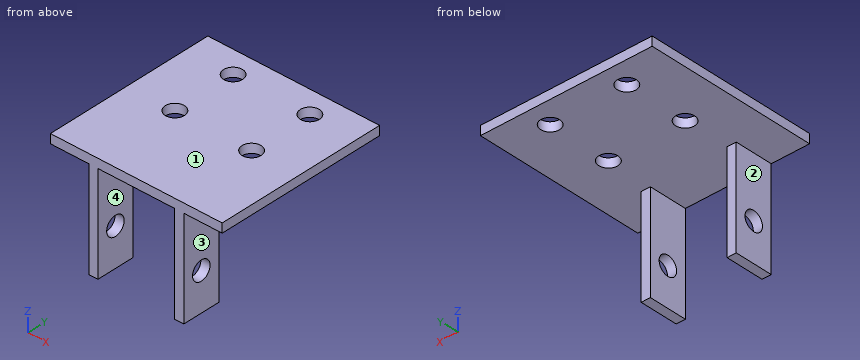
Autodesk Fusion 360 part; units mm, degrees
sketch "Sketch1" plane through (0, 0, 0) normal (0, 0, 1) x (1, 0, 0)
  line L0 (-13.45, 12) -> (31.55, 12)
  line L1 (31.55, 12) -> (31.55, -33)
  line L2 (31.55, -33) -> (-13.45, -33)
  line L3 (-13.45, -33) -> (-13.45, 12)
  line L4 (-3.4, -33) -> (-1, -33)
  line L5 (-1, -33) -> (-1, -23)
  line L6 (-1, -23) -> (-3.4, -23)
  line L7 (-3.4, -23) -> (-3.4, -33)
  line L8 (19.1, -23) -> (19.1, -33)
  line L9 (21.5, -23) -> (19.1, -23)
  line L10 (21.5, -33) -> (21.5, -23)
  line L11 (19.1, -33) -> (21.5, -33)
  circle A0 centre (-1, 5.65) radius 2.5
  circle A1 centre (-1, 5.65) radius 7.65
  circle A2 centre (19.1, 5.65) radius 7.65
  circle A3 centre (19.1, 5.65) radius 2.5
  circle A4 centre (-1, -11) radius 2.5
  circle A5 centre (19.1, -11) radius 2.5
  circle A6 centre (-1, -11) radius 9
  circle A7 centre (19.1, -11) radius 9
  dimension "d1" = 45
  dimension "d2" = 45
  dimension "d3" = 10
  dimension "d4" = 2.4
  dimension "d5" = 10.05
  dimension "d7" = 2.4
  dimension "d8" = 20.1
  dimension "d9" = 5
  dimension "d10" = 6.35
  dimension "d11" = 15.3
  dimension "d13" = 5
  dimension "d14" = 15.3
  dimension "d15" = 20.1
  dimension "d16" = 12.45
  dimension "d25" = 5
  dimension "d26" = 5
  dimension "d27" = 20.1
  dimension "d28" = 12.45
  dimension "d31" = 18
  dimension "d32" = 18
extrude "Extrude1" add sketch "Sketch1" along normal blind 2.4 contours A7 | A6 | L0 L1 L2 L3 L5 L6 L7 L8 L9 L10 A1 A2 | L0 A1 | L2 L4 L5 L6 L7 | L0 A2 | L2 L8 L9 L10 L11 | A4 | A5 picked at (-1.0623, 10.7143) picked at (19.0377, 10.7143)
extrude "Extrude2" add sketch "Sketch1" against normal blind 26 contours L2 L4 L5 L6 L7 | L2 L8 L9 L10 L11
sketch "Sketch2" plane through (21.5, 0, 0) normal (1, 0, 0) x (0, 1, 0)
  line L0 (-23, 0) -> (-33, 0)
  line L1 (-33, 0) -> (-33, -26)
  line L2 (-33, -26) -> (-23, -26)
  line L3 (-23, -26) -> (-23, 0)
  circle A0 centre (-28, -16) radius 2.5
  dimension "d21" = 5
  dimension "d22" = 10
extrude "Extrude3" cut sketch "Sketch2" against normal blind 30 contours A0
extrude "Extrude4" cut sketch "Sketch1" along normal blind 3 contours A4 | A5
Geometry: final body of the model. Coordinates: model frame, mm. Face numbers are marked on the shaded views. Round coordinates to 2 decimals unless told otherwise and drop trailing zeros. Write each loop counter-clockwise with the first axis right and the second up, starting at its lowest first coordinate (ties: lowest second). Pieces come first, ordered by that corner, then holes. Notation, with made-up numbers: M -16,-18.5 L -6,-18.5 A25 ccw -6,9.5 Z; hole C -32,31 d2. An arc over 180 degrees is marked long. Answer in a Markdown table with one row per item. Add a question column.
(1) Cut plane C-C, the plane z = -16. Return the cut outline in (x, y).
(2) Ray query, L1, parallel to X at y = -11, z = 1.8; L2, parallel to Y at x = 19.1, z = 0.7; L3, parallel to Z at x = -2.05, y = -28. Return the intervals inside material, ascending.
(3) Cut plane D-D, the plane y = -12.5. Return the cut outline in (x, z).
(4) Contact query for flat-ended pins moving along their axis: pin 1 (6 mm diameter, centred on x = -1, y = -11, fed in from -Z); pin 2 (8 mm diameter, centred on y = -28, z = -16, fed in from +X); pin 3 (6 mm diameter, centred on y = -28, z = -16, fed in from -X); pin 4 (4 mm diameter, centred on x = 19.1, y = -11, fed in from +Z). Output: stop coordinate, or through.
(5) Cut plane B-B, the plane z = -7.75. Return the cut outline in (x, y), then the cut area to 3 significant figures.
(6) Draft query along X for the marked faces 1, 2, 3 and 4. Return one class per face: pulls with the +X half, pulls with the -X half, needs draft (parallel to the pull), parting line crosses it, or undercut.
(7) Cut plane A-A, the plane y = -28. Return the cut outline in (x, z), then the cut area to 3 significant figures.
Established:
| question | item | result |
|---|---|---|
| 1 | outline | M -3.4,-33 L -1,-33 L -1,-30.5 L -3.4,-30.5 Z; M -3.4,-25.5 L -1,-25.5 L -1,-23 L -3.4,-23 Z; M 19.1,-33 L 21.5,-33 L 21.5,-30.5 L 19.1,-30.5 Z; M 19.1,-25.5 L 21.5,-25.5 L 21.5,-23 L 19.1,-23 Z |
| 2 | L1 | -13.45 to -3.5, 1.5 to 16.6, 21.6 to 31.55 |
| 2 | L2 | -33 to -13.5, -8.5 to 3.15, 8.15 to 12 |
| 2 | L3 | -26 to -18.5, -13.5 to 2.4 |
| 3 | outline | M -13.45,0 L -3,0 L -3,2.4 L -13.45,2.4 Z; M 1,0 L 17.1,0 L 17.1,2.4 L 1,2.4 Z; M 21.1,0 L 31.55,0 L 31.55,2.4 L 21.1,2.4 Z |
| 4 | pin 1 | z = 0 |
| 4 | pin 2 | x = 21.5 |
| 4 | pin 3 | x = -3.4 |
| 4 | pin 4 | through |
| 5 | outline | M -3.4,-33 L -1,-33 L -1,-23 L -3.4,-23 Z; M 19.1,-33 L 21.5,-33 L 21.5,-23 L 19.1,-23 Z |
| 5 | area | 48.0 mm² |
| 6 | face 1 | needs draft |
| 6 | face 2 | pulls with the -X half |
| 6 | face 3 | pulls with the +X half |
| 6 | face 4 | undercut |
| 7 | outline | M -13.45,0 L -3.4,0 L -3.4,-13.5 L -1,-13.5 L -1,0 L 19.1,0 L 19.1,-13.5 L 21.5,-13.5 L 21.5,0 L 31.55,0 L 31.55,2.4 L -13.45,2.4 Z; M -3.4,-26 L -1,-26 L -1,-18.5 L -3.4,-18.5 Z; M 19.1,-26 L 21.5,-26 L 21.5,-18.5 L 19.1,-18.5 Z |
| 7 | area | 209 mm² |
